The listing builds one solid part. Answer for the finished solid, in the listing's coordinates (mm). A direction names the side the tool comes from. Round coordinates to 2 decimals unless told otherwise and drop trailing zeros. Write each loop counter-clockwise with the first axis right and the second up, starting at its lowest first coordinate (ties: lowest second). Pieces come first, ordered by that corner, then holes.
(1) Each of these flat-tipped pins is pushed along its axis until it touches: pin 1 Ø20.5 at (x, y) = (-483, -12) entering from -Z; pin 2 Ø7.5 at (x, y) = (-473, -11) entering from +Z; pin 3 Ø3 at (x, z) = (-369.5, -385.5) entering from -Y. Where does it stop, or does it pass through?
(2) A cutting plane is placed at C-C, the plane x = -317. Give the vertices of the cut face in (y, z).
(3) Find the intervals of material crossed by probe 1 along Z at (x, y) = (-446, -20.5); probe 2 along Y at (x, z) = (-153, -625); probe 3 along Z at (x, y) = (-194, 0.5), in increasing order.
(4) For faces 5 (the face through (-477, -13, -381)), 6 (the face through (-444.5, -13, -1080)), 7 (the face through (-250, 38.1, -751)), 8 (the face through (-477, -13, -1143)), determine the directions among +Z, -Z, +X, -X, +Y, -Y from which every point of the face is accessible in a straight line to the end or side of a thin tool.
(5) A cutting plane is placed at D-D, the plane x = -233.5. Give the vertices of the cut face in (y, z), and give its area (3 significant figures).
(6) The mould has two halves that part along Z. Classify faces 1 (the face through (-477, -25.4, -1079)), 2 (the face through (-476, -13, -508)), 3 (the face through (-476, -13, -1016)), 4 (the face through (-72.43, 19.32, -1447.62)): +Z half, -Z half, draft (parallel to the pull), parting line (faces both ways), or undercut.
(7) A cutting plane is placed at B-B, the plane z = -1041. Give the vertices of the cut face in (x, y), and give its area (3 significant figures).
(8) A cutting plane is placed at A-A, the plane y = -14. Give the vertices of the cut face in (x, z), and give its area (3 significant figures).
Autodesk Inventor part; units mm, degrees
ref_plane "YZ Plane" through (0, 0, 0) normal (1, 0, 0) x (0, 1, 0)
ref_plane "XZ Plane" through (0, 0, 0) normal (0, 1, 0) x (-1, 0, 0)
ref_plane "XY Plane" through (0, 0, 0) normal (0, 0, 1) x (1, 0, 0)
sketch "Sketch1" plane through (0, 0, 0) normal (0, 1, 0) x (-1, 0, 0)
  line L0 (0, 0) -> (508, 0)
  line L1 (508, 0) -> (508, -1524)
  line L2 (508, -1524) -> (0, -1524)
  line L3 (0, -1524) -> (0, 0)
  dimension "d0" = 1524
  dimension "d1" = 508
extrude "Extrusion1" add sketch "Sketch1" along normal blind 38.1
fillet "Fillet1" radius 254 1 edges at (0, 19.05, 0)
fillet "Fillet2" radius 254 1 edges at (0, 19.05, -1524)
sketch "Sketch2" plane through (0, 0, 0) normal (0, -1, 0) x (1, 0, 0)
  line L0 (-254, -1524) -> (-508, -1524)
  line L1 (-508, -1524) -> (-508, 0)
  line L2 (-508, -1524) -> (-508, 0)
  line L3 (-508, 0) -> (-508, -381)
  line L4 (-508, -381) -> (-444.5, -381)
  line L5 (-444.5, -381) -> (-444.5, -508)
  line L6 (-444.5, -508) -> (-508, -508)
  line L7 (-508, -1524) -> (-508, -1143)
  line L8 (-508, -1143) -> (-444.5, -1143)
  line L9 (-444.5, -1143) -> (-444.5, -1016)
  line L10 (-444.5, -1016) -> (-508, -1016)
  point P0 (0, 0)
  dimension "d6" = 381
  dimension "d7" = 63.5
  dimension "d8" = 127
  dimension "d9" = 381
  dimension "d10" = 127
extrude "Extrusion2" add sketch "Sketch2" along normal blind 25.4
properties part number "Shelf-ver1-1111-2021" material "Aluminum 6061"
Solutions:
1. pin 1: stops at z = -1143
1. pin 2: stops at z = -381
1. pin 3: stops at y = 0
2. outline: (0, -1524) - (38.1, -1524) - (38.1, 0) - (0, 0) - close
3. probe 1: z = -1143 to -1016, -508 to -381
3. probe 2: y = 0 to 38.1
3. probe 3: z = -1516.81 to -7.19
4. face 5: +Z, +X, -X, -Y
4. face 6: +Z, -Z, +X, -Y
4. face 7: +Z, -Z, +X, -X, +Y
4. face 8: -Z, +X, -X, -Y
5. outline: (0, -1523.17) - (38.1, -1523.17) - (38.1, -0.83) - (0, -0.83) - close
5. area: 58,000 mm2
6. face 1: draft
6. face 2: undercut
6. face 3: undercut
6. face 4: -Z half
7. outline: (-508, -25.4) - (-444.5, -25.4) - (-444.5, 0) - (0, 0) - (0, 38.1) - (-508, 38.1) - close
7. area: 21,000 mm2
8. outline: (-508, -1143) - (-444.5, -1143) - (-444.5, -1016) - (-508, -1016) - close; (-508, -508) - (-444.5, -508) - (-444.5, -381) - (-508, -381) - close
8. area: 16,100 mm2
